```python
from build123d import *


with BuildPart() as part:
    # Sketch → Revolution (revolve)
    with BuildSketch(Plane.XY):
        with BuildLine():
            Line((17.677678, -954.92), (232.322322, -954.92))
            Line((232.322322, -954.92), (250, -972.597661))
            Line((250, -1008.225592), (250, -972.597661))
            ThreePointArc((232.40613, -1034.220062), (245.188053, -1023.919992), (250, -1008.225592))
            ThreePointArc((17.59387, -1034.220062), (125, -1054.92), (232.40613, -1034.220062))
            ThreePointArc((0, -1008.225592), (4.811947, -1023.919992), (17.59387, -1034.220062))
            Line((0, -972.597661), (0, -1008.225592))
            Line((17.677678, -954.92), (0, -972.597661))
        make_face()
    revolve(axis=Axis((0, 0, 0), (1, 0, 0)))


solid = part.part
```
Can you work these out from the model? Positions are in its coordinate system, mm. Coordinates: 2 decimals unless noted, no trailing zeros. Order: outer loops, then holes, each group sorted by start corner. A loop starts at its lowest first (then second) coordinate and runs counter-clockwise, first axis right, second up.
1. If we section it at A-A (y = 0): Please give me the cut outline in (x, z), then the cut area to 3 significant figures.
2. If we section it at C-C (x = 116.5): Please give me the cut outline in (y, z), then the cut area to 3 significant figures.
3. Thinking about a two-plate mould opening in Y: for faces 1 (the face through (0, -527, -826)), 2 (the face through (126.503, 757.792, 581.054)), which applies, +Y half, -Y half, draft (parallel to the pull), parting line (faces both ways), or undercut?
4. I need wall thicknesses on line 1 (Z direction, x = 140, y = 0); line 2 (Z direction, x = 134.5, y = 0); line 3 (Y direction, x = 67, z = -465). Which ranges of each line are inside material? Lowest first, please.
5. I'm going to push flat-ended pins straight in: pin 1 (10 mm diameter, centred on x = 204.5, y = 700.5, fed in from -Z); pin 2 (4 mm diameter, centred on x = 114.5, z = -158, fed in from -Y); pin 3 (10 mm diameter, centred on x = 63, y = -685.5, fed in from +Z). Where does each tip first touch, or does it pass through?
Entries:
1. outline: (0, -1008.23) arc R28 ccw to (17.59, -1034.22) arc R289 ccw to (232.41, -1034.22) arc R28 ccw to (250, -1008.23) - (250, -972.6) - (232.32, -954.92) - (17.68, -954.92) - (0, -972.6) - close; (0, 972.6) - (17.68, 954.92) - (232.32, 954.92) - (250, 972.6) - (250, 1008.23) arc R28 ccw to (232.41, 1034.22) arc R289 ccw to (17.59, 1034.22) arc R28 ccw to (0, 1008.23) - close
1. area: 44,500 mm2
2. outline: circle Ø2109.59 at (0, 0); hole circle Ø1909.84 at (0, 0)
2. area: 631,000 mm2
3. face 1: draft
3. face 2: undercut
4. line 1: z = -1054.53 to -954.92, 954.92 to 1054.53
4. line 2: z = -1054.76 to -954.92, 954.92 to 1054.76
4. line 3: y = -940.35 to -834.05, 834.05 to 940.35
5. pin 1: stops at z = -778.68
5. pin 2: stops at y = -1043.14
5. pin 3: stops at z = 797.49
